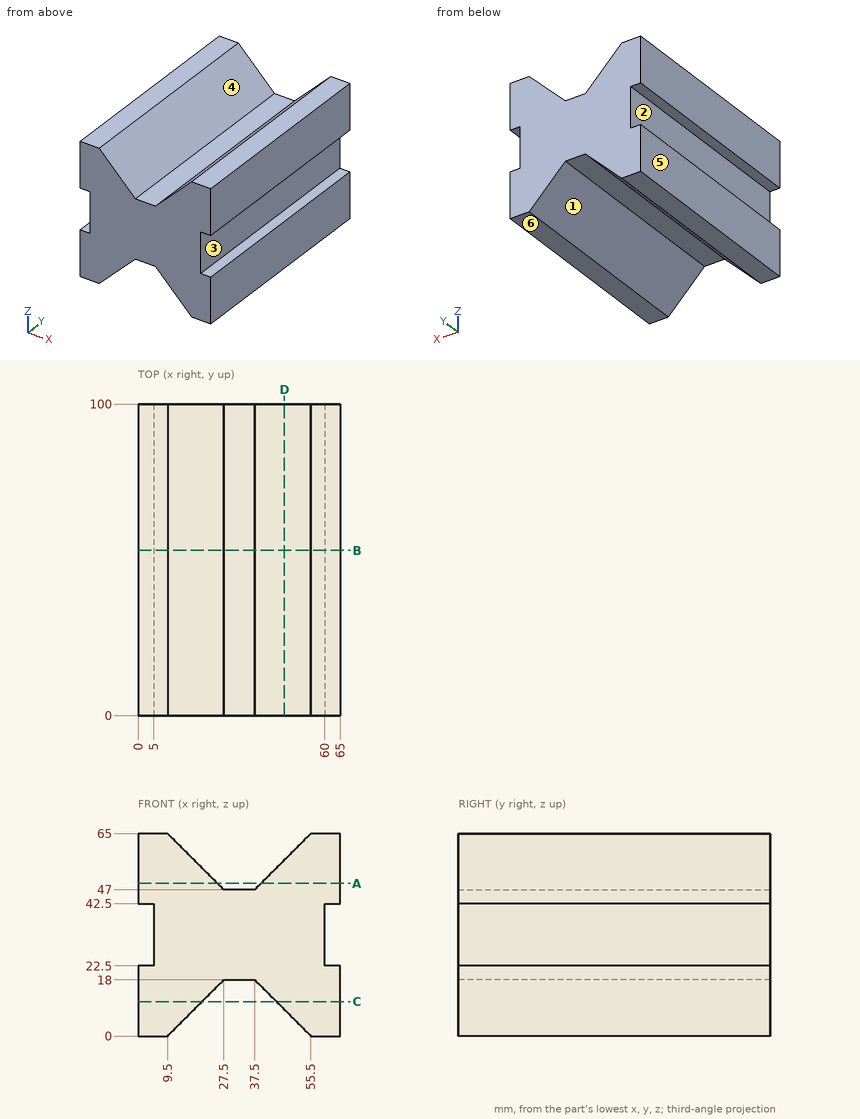
Geometry check sheet. Reference: drawing and pictorial views, mm from the part's lowest x, y, z. A direction names the side the tool comes from. Give positions to 0.01 mm unless a question says otherwise; leave off trailing zeros. Write each loop counter-clockwise with the first axis right and the second up, starting at its lowest first coordinate (ties: lowest second). Pieces come first, ordered by that corner, then holes.
Item 1: Scan lines: L1, parallel to X at y = 20.5, z = 56.5; L2, parallel to Z at x = 36.5, y = 38.5; L3, parallel to X at y = 25, z = 27. Record each from-to range of solid material in increasing order.
Item 2: Cross-section at A-A (z = 49). Enter the section's corners in (x, y).
Item 3: Draft check along X on the marked faces 4, 5 and 6. Enter one of: released by +X, released by -X, zero draft, split by the parting line, or undercut.
Item 4: Gauge pin test, flat ends, axial feed: pin 1 (3 mm diameter, centred on x = 34.5, y = 55, fed in from -Z); pin 2 (10 mm diameter, centred on y = 37, z = 28.5, fed in from +X); pin 3 (6 mm diameter, centred on y = 52, z = 34, fed in from -X). Record the tip position at first contact, or that the pin passes through.
Item 5: Cross-section at D-D (x = 47). Enter the section's corners in (y, z), and give its area (3 significant figures).
Item 6: Access from +Z, -Z, +X, -X, +Y, -Y to the whole of each face (thin tool, end or side, straight path). Record for the marked faces 1, 2 and 3.
Item 7: Cross-section at C-C (z = 11). Enter the section's corners in (x, y).
Item 8: Cross-section at B-B (y = 53). Enter the section's corners in (x, z), and give its area (3 significant figures).
Report:
1. L1: x = 0 to 18, 47 to 65
1. L2: z = 18 to 47
1. L3: x = 5 to 60
2. outline: (0, 0) - (25.5, 0) - (25.5, 100) - (0, 100) - close; (39.5, 0) - (65, 0) - (65, 100) - (39.5, 100) - close
3. face 4: undercut
3. face 5: released by -X
3. face 6: zero draft
4. pin 1: stops at z = 18
4. pin 2: stops at x = 60
4. pin 3: stops at x = 5
5. outline: (0, 8.5) - (100, 8.5) - (100, 56.5) - (0, 56.5) - close
5. area: 4,800 mm2
6. face 1: -Z, +Y, -Y
6. face 2: -X, +Y, -Y
6. face 3: +X, +Y, -Y
7. outline: (0, 0) - (20.5, 0) - (20.5, 100) - (0, 100) - close; (44.5, 0) - (65, 0) - (65, 100) - (44.5, 100) - close
8. outline: (0, 0) - (9.5, 0) - (27.5, 18) - (37.5, 18) - (55.5, 0) - (65, 0) - (65, 22.5) - (60, 22.5) - (60, 42.5) - (65, 42.5) - (65, 65) - (55.5, 65) - (37.5, 47) - (27.5, 47) - (9.5, 65) - (0, 65) - (0, 42.5) - (5, 42.5) - (5, 22.5) - (0, 22.5) - close
8. area: 3,020 mm2
